```python
from build123d import *

# Parameters (mm, degrees)
SKETCH1_R           = 5
BOSS_EXTRUDE1_DEPTH = 10
CHAMFER1_SIZE       = 3


with BuildPart() as part:
    # Sketch1 → Boss-Extrude1 (new body)
    with BuildSketch(Plane(origin=(0, 0, 0), x_dir=(1, 0, 0), z_dir=(0, 1, 0))):
        with BuildLine():
            Line((-4.472135955, 27.763932023), (-42.11145618, 8.94427191))
            ThreePointArc((-42.11145618, 8.94427191), (-47.639320225, 0), (-42.11145618, -8.94427191))
            Line((-42.11145618, -8.94427191), (-4.472135955, -27.763932023))
            ThreePointArc((-4.472135955, -27.763932023), (0, -28.819660113), (4.472135955, -27.763932023))
            Line((4.472135955, -27.763932023), (42.11145618, -8.94427191))
            ThreePointArc((42.11145618, -8.94427191), (47.639320225, 0), (42.11145618, 8.94427191))
            Line((42.11145618, 8.94427191), (4.472135955, 27.763932023))
            ThreePointArc((4.472135955, 27.763932023), (0, 28.819660113), (-4.472135955, 27.763932023))
        make_face()
        with Locations(Location((0, 18.819660113, 0), (0, 0, 270))):
            Circle(SKETCH1_R, mode=Mode.SUBTRACT)
        with Locations(Location((37.639320225, 0, 0), (0, 0, 270))):
            Circle(SKETCH1_R, mode=Mode.SUBTRACT)
        with Locations(Location((0, -18.819660113, 0), (0, 0, 270))):
            Circle(SKETCH1_R, mode=Mode.SUBTRACT)
        with Locations(Location((-37.639320225, 0, 0), (0, 0, 270))):
            Circle(SKETCH1_R, mode=Mode.SUBTRACT)
    extrude(amount=BOSS_EXTRUDE1_DEPTH)

    # Chamfer1
    chamfer1_edges = [part.edges().sort_by_distance(p)[0] for p in [
        (0, 0, -23.819660113),
        (0, 10, -23.819660113),
        (37.639320225, 0, -5),
        (37.639320225, 10, -5),
        (0, 0, 13.819660113),
        (0, 10, 13.819660113),
        (-37.639320225, 0, -5),
        (-37.639320225, 10, -5),
    ]]
    chamfer(chamfer1_edges, length=CHAMFER1_SIZE)


solid = part.part
```
Check sheet for the modelled part. Datum: model origin and axes. Units: mm. Coordinates: 2 decimals unless noted, no trailing zeros. Write each loop counter-clockwise with the first axis right and the second up, starting at its lowest first coordinate (ties: lowest second). Pieces come first, ordered by that corner, then holes. Notation, with made-up numbers: M -27,-1.5 L 18,-1.5 A19 ccw 18,15.5 Z; hole C 9,1 d11. An arc over 180 degrees is marked long. Write item = value, one per line. Start each with the question number.
1. Sectioned sample at B-B (z = 0). Record the cut outline in (x, y).
2. Sectioned sample at C-C (y = 1.5). Record the cut outline in (x, z), then the cut area to 3 significant figures.
3. Go/stop test with flat-tipped pins: pin 1 (6 mm diameter, centred on x = 6, z = 15.5, fed in from -Y); pin 2 (1.5 mm diameter, centred on x = -21.5, y = 4, fed in from -Z) (3 decimals); pin 3 (5 mm diameter, centred on y = 2, z = 15.5, fed in from -X); pin 4 (1.5 mm diameter, centred on y = 1.5, z = -3.5, fed in from +X). Record where each tip stops, or that it passes through.
4. Mould release check, pull along Z, two halves, no side actions. Record for faces 1 (the cylindrical face through (47.64, 4.93, 0.15)), 2 (the flat face through (-24, 5, 18)), 3 (the conical face through (-42.242, 2.812, 2.394)), 4 (the flat face through (-1, 0, 0)): pulls with the +Z half, pulls with the -Z half, needs draft (parallel to the pull), parting line crosses it, or undercut.
5. Sectioned sample at D-D (x = -10.5). Record the cut outline in (y, z), then the cut area to 3 significant figures.
6. Thickness scan on probe 1 along X at (y, z) = (2, 5); probe 2 along X at (y, z) = (1.5, 4); probe 3 along Z at (x, y) = (4, 4.5). Record the ranges inside material, lowest first.
7. Sectioned sample at A-A (x = 0). Record the cut outline in (y, z).
The answers:
q1.outline = M -47.64,0 L -45.64,0 L -42.64,3 L -42.64,7 L -45.64,10 L -47.64,10 Z; M -32.64,3 L -29.64,0 L 29.64,0 L 32.64,3 L 32.64,7 L 29.64,10 L -29.64,10 L -32.64,7 Z; M 42.64,3 L 45.64,0 L 47.64,0 L 47.64,10 L 45.64,10 L 42.64,7 Z
q2.outline = M -42.11,-8.94 L -4.47,-27.76 A10 ccw 4.47,-27.76 L 42.11,-8.94 A10 ccw 42.11,8.94 L 4.47,27.76 A10 ccw -4.47,27.76 L -42.11,8.94 A10 ccw Z; hole C -37.64,0 d13; hole C 0,-18.82 d13; hole C 0,18.82 d13; hole C 37.64,0 d13
q2.area = 2,880 mm²
q3.pin_1 = 0
q3.pin_2 = -19.625
q3.pin_3 = -34
q3.pin_4 = 47.25
q4.face_1 = parting line crosses it
q4.face_2 = pulls with the +Z half
q4.face_3 = undercut
q4.face_4 = needs draft
q5.outline = M 0,-24.75 L 10,-24.75 L 10,24.75 L 0,24.75 Z
q5.area = 495 mm²
q6.probe_1 = -46.3 to -40.96, -34.32 to 34.32, 40.96 to 46.3
q6.probe_2 = -46.8 to -42.76, -32.52 to 32.52, 42.76 to 46.8
q6.probe_3 = -27.98 to -21.82, -15.82 to 15.82, 21.82 to 27.98
q7.outline = M 0,-28.82 L 10,-28.82 L 10,-26.82 L 7,-23.82 L 3,-23.82 L 0,-26.82 Z; M 0,-10.82 L 3,-13.82 L 7,-13.82 L 10,-10.82 L 10,10.82 L 7,13.82 L 3,13.82 L 0,10.82 Z; M 0,26.82 L 3,23.82 L 7,23.82 L 10,26.82 L 10,28.82 L 0,28.82 Z
